Geometry check sheet. Reference: drawing and pictorial views, mm from the part's lowest x, y, z. Give positions to 0.01 mm unless a question says otherwise; leave off trailing zeros. Write each loop counter-clockwise with the first axis right and the second up, starting at its lowest first coordinate (ties: lowest second). Pieces come first, ordered by that corner, then holes. Notation, with made-up numbers: (23, 83) - (65, 83) arc R19 ccw to (65, 97) - close; hole circle Ø1 at (19.25, -28.5). An arc over 180 degrees is marked (long way). Write item = value, one per line. Start each with the question number.
(1) Depth check by flat-ended pin: pin 1 Ø5 at (x, z) = (85.725, 44.45) entering from +Y; pin 2 Ø2 at (x, z) = (156, 220) entering from -Y. Enter the tip coordinate at first touch or a pass-through.
(2) Section check B-B, the plane x = 57.15. Enter the section's corners in (y, z), plus the area to 3 significant figures.
(3) Section check C-C, the plane y = 3.95. Give the number of separate pieces and of enclosed holes in the cut face, plus the area to 3 significant figures.
(4) Thickness scan on L1, parallel to X at y = 4.3, z = 190.5; L2, parallel to Z at x = 349.25, y = 3.65; L3, parallel to Z at x = 40.5, y = 2.55. Record the ranges inside material, lowest first.
(5) Section check A-A, the plane z = 223. Enter the section's corners in (x, y), plus the area to 3 significant figures.
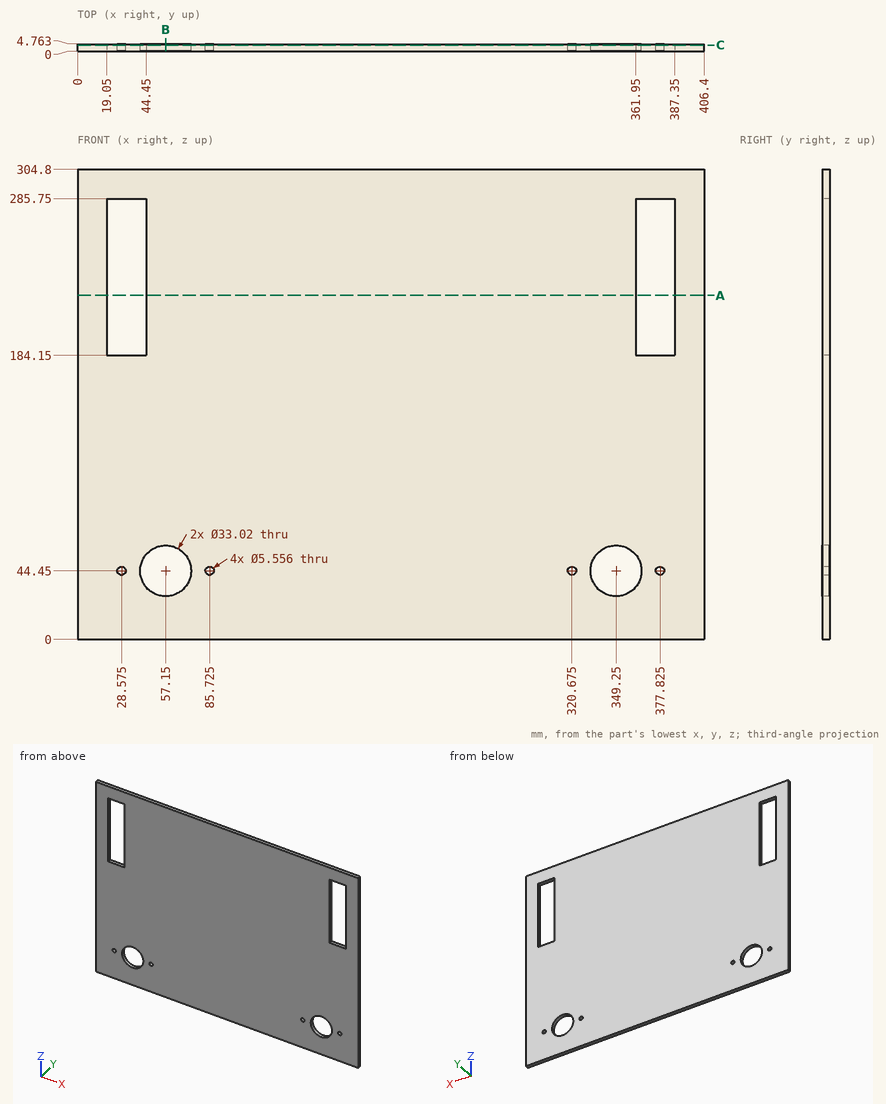
Model answer:
q1.pin_1 = through
q1.pin_2 = 0
q2.outline = (0, 0) - (4.76, 0) - (4.76, 27.94) - (0, 27.94) - close; (0, 60.96) - (4.76, 60.96) - (4.76, 304.8) - (0, 304.8) - close
q2.area = 1,290 mm²
q3.separate_pieces = 1
q3.enclosed_holes = 8
q3.area = 117,000 mm²
q4.L1 = 0 to 19.05, 44.45 to 361.95, 387.35 to 406.4
q4.L2 = 0 to 27.94, 60.96 to 304.8
q4.L3 = 0 to 184.15, 285.75 to 304.8
q5.outline = (0, 0) - (19.05, 0) - (19.05, 4.76) - (0, 4.76) - close; (44.45, 0) - (361.95, 0) - (361.95, 4.76) - (44.45, 4.76) - close; (387.35, 0) - (406.4, 0) - (406.4, 4.76) - (387.35, 4.76) - close
q5.area = 1,690 mm²
